Read the model definition and answer for the solid it produces. Units are mm, in the model's axes. A direction names the side the tool comes from. Round coordinates to 2 decimals unless told otherwise and drop trailing zeros. Loops run counter-clockwise (first coordinate to the right, second up) from the corner with the lowest first, then second, coordinate; pieces in that order, holes last. Notation, with made-up numbers: M 70,-31.5 L 120,-31.5 A20 cw 120,5.5 Z; hole C 58,18.5 d7. An arc over 180 degrees is marked long. Write each question's results on one line, items separated by ' | '.
Autodesk Inventor part; units mm, degrees
ref_plane "YZ Plane" through (0, 0, 0) normal (1, 0, 0) x (0, 1, 0)
ref_plane "XZ Plane" through (0, 0, 0) normal (0, 1, 0) x (-1, 0, 0)
ref_plane "XY Plane" through (0, 0, 0) normal (0, 0, 1) x (1, 0, 0)
sketch "Sketch1" plane through (0, 0, 0) normal (0, 0, 1) x (1, 0, 0)
  line L0 (-12.5, -17.5) -> (12.5, -17.5)
  line L1 (12.5, -17.5) -> (12.5, 17.5)
  line L2 (-12.5, 17.5) -> (-12.5, -17.5)
  line L3 (12.5, 17.5) -> (-12.5, 17.5)
  circle A0 centre (0, 0) radius 2.05
  dimension "d0" = 4.1
extrude "Extrusion1" add sketch "Sketch1" along normal blind 7
sketch "Sketch2" plane through (0, 0, 0) normal (0, 0, -1) x (-1, 0, 0)
  circle A0 centre (-8, -12) radius 2.1
  circle A1 centre (7, 12) radius 2.1
  circle A2 centre (-8, -12) radius 1.9
  circle A3 centre (7, 12) radius 1.9
  dimension "d9" = 3.8
extrude "Extrusion3" add sketch "Sketch2" along normal blind 6 draft -1 contours A2 | A3
sketch "Sketch3" plane through (0, 0, 0) normal (0, 0, -1) x (-1, 0, 0)
  line L0 (5.5902, -5) -> (-5.5902, -5) construction
  line L1 (-5.5902, 5) -> (5.5902, 5) construction
  line L2 (-7, -5.2) -> (7, -5.2)
  line L3 (7, -5.2) -> (7, 5.2)
  line L4 (7, 5.2) -> (-7, 5.2)
  line L5 (-7, 5.2) -> (-7, -5.2)
  line L6 (-6, -4.5) -> (-6, 4.5) construction
  line L7 (6, 4.5) -> (6, -4.5) construction
  line L8 (-5.5902, 5) -> (5.5902, 5)
  line L9 (5.5902, -5) -> (-5.5902, -5)
  dimension "d28" = 1
  dimension "d29" = 1
  dimension "d30" = 0.2
  dimension "d31" = 0.2
extrude "Extrusion4" cut sketch "Sketch3" against normal blind 5.2
sketch "Sketch4" plane through (0, 0, 5.2) normal (0, 0, -1) x (-1, 0, 0)
  circle A0 centre (-4.5, 0) radius 0.6105
  circle A1 centre (4.5, 0) radius 0.6105
  circle A2 centre (-4.5, 0) radius 0.5
  circle A3 centre (4.5, 0) radius 0.5
  point P0 (0, 0)
  dimension "d18" = 1
extrude "Extrusion5" add sketch "Sketch4" along normal blind 2 contours A2 | A3
fillet "Fillet1" radius 0.2 2 edges at (-4, 0, 5.2) (5, 0, 5.2)
fillet "Fillet2" radius 0.4 2 edges at (-4, 0, 3.2) (5, 0, 3.2)
fillet "Fillet3" radius 0.5 2 edges at (-5.1, 12, 0) (9.9, -12, 0)
properties part number "Base-Cover" material "Polycarbonate, Clear"
Item 1: Straight lines are drawn through the part: line 1 (X direction, y = -5, z = 0.75); line 2 (Y direction, x = -2.5, z = 3); line 3 (Y direction, x = 0, z = 6.6). For each, find the intervals that lie inside material, in ascending order.
Outcome:
line 1: x = -12.5 to -7, 7 to 12.5 | line 2: y = -17.5 to -5.2, 5.2 to 17.5 | line 3: y = -17.5 to -2.05, 2.05 to 17.5
Item 2: Flat-ended cylindrical pins translate along their axes: pin 1 (12 mm diameter, centred on x = 4, y = -3.5, fed in from -Z); pin 2 (4.5 mm diameter, centred on x = 0, y = 0, fed in from -Z). Find the tip coordinate at first contact, or state that the pin passes through.
Outcome:
pin 1: stops at z = 0 | pin 2: stops at z = 5.2
Item 3: The part is cut by section C-C (z = -3.5). Determine the outline of the cut face in (x, y).
Outcome:
outline: C -7,12 d3.68; C 8,-12 d3.68
Item 4: The part is cut by section A-A (x = 0). Determine the outline of the cut face in (y, z).
Outcome:
outline: M -17.5,0 L -5.2,0 L -5.2,5.2 L -2.05,5.2 L -2.05,7 L -17.5,7 Z; M 2.05,5.2 L 5.2,5.2 L 5.2,0 L 17.5,0 L 17.5,7 L 2.05,7 Z
Item 5: The mould has two halves that part along Y. Classify faces 3 (the face through (0, -17.5, 3)), 4 (the face through (8, -12, -6)), 5 (the face through (0, -5.2, 3)): pulls with the +Y half, pulls with the -Y half, needs draft (parallel to the pull), parting line crosses it, or undercut.
Outcome:
face 3: pulls with the -Y half | face 4: needs draft | face 5: undercut
Item 6: For faces 1 (the face through (7, 0, 3)), 2 (the face through (-12.5, 0, 3)), determine the directions among +Z, -Z, +X, -X, +Y, -Y from which every point of the face is accessible in a straight line to the end or side of a thin tool.
Outcome:
face 1: -Z | face 2: +Z, -Z, -X, +Y, -Y
Item 7: The part is cut by section B-B (y = 4.5). Determine the outline of the cut face in (x, z), plus the area to 3 significant figures.
Outcome:
outline: M -12.5,0 L -7,0 L -7,5.2 L 7,5.2 L 7,0 L 12.5,0 L 12.5,7 L -12.5,7 Z | area: 102 mm2
